Design review of the part built by this model. Coordinates are the model's own, in mm. A direction names the side the tool comes from. Coordinates: 2 decimals unless noted, no trailing zeros. Order: outer loops, then holes, each group sorted by start corner. A loop starts at its lowest first (then second) coordinate and runs counter-clockwise, first axis right, second up. Notation, with made-up numbers: (-12, -21.75) -> (44, -21.75) arc R25 cw to (44, -2.75) -> close; hole circle Ø4 at (44.25, 55.25). An arc over 180 degrees is marked (long way). Write item = value, one per line.
```python
from build123d import *

# Parameters (mm, degrees)
SKETCH1_R           = 2.75
BOSS_EXTRUDE1_DEPTH = 3.2


with BuildPart() as part:
    # Sketch1 → Boss-Extrude1 (new body)
    with BuildSketch(Plane.XY):
        Polygon((0, 82), (0, 3), (3, 0), (82, 0), (85, 3), (85, 15), (82, 18), (18, 18), (18, 82), (15, 85), (3, 85), align=None)
        with Locations((75, 9)):
            Circle(SKETCH1_R, mode=Mode.SUBTRACT)
        with Locations((47, 9)):
            Circle(SKETCH1_R, mode=Mode.SUBTRACT)
        with Locations((9, 47)):
            Circle(SKETCH1_R, mode=Mode.SUBTRACT)
        with Locations((9, 75)):
            Circle(SKETCH1_R, mode=Mode.SUBTRACT)
    extrude(amount=-BOSS_EXTRUDE1_DEPTH)


solid = part.part
```
(1) The part is to be moulded in two halves that separate along Y. For faces 3 (the cylindrical face through (8.642, 49.727, -1.578)), 4 (the cylindrical face through (8.642, 77.727, -1.578)), 5 (the flat face through (2, 84, -2)), 6 (the flat face through (83, 1, -2)), say which applies: released by +Y, released by -Y, zero draft, split by the parting line, or undercut.
Report:
face_3 = undercut
face_4 = undercut
face_5 = released by +Y
face_6 = released by -Y
(2) Insertion check: pin 1 (1.6 mm diameter, centred on y = 47.5, z = -2, fed in from +X); pin 2 (1 mm diameter, centred on x = 26.5, z = -2.5, fed in from +Y); pin 3 (1.5 mm diameter, centred on x = 22, z = -2, fed in from -Y). Each pin has a flat end and moves straight along its axis. Give the tip position at first contact, or say it passes through.
Report:
pin_1 = 18
pin_2 = 18
pin_3 = 0
(3) For faces 1 (the flat face through (50, 18, -2)), 2 (the cylindrical face through (72.253, 9.121, -1.578)), list the 3-axis set-ups (+Z, -Z, +X, -X, +Y, -Y) from which the entire face can be reached by the end or side of a thin tool; tool diameter is ignored.
Report:
face_1 = +Z, -Z, +X, +Y
face_2 = +Z, -Z
(4) We need section A-A (y = 9). Write out the cut boundary in (x, z), and give its area (3 significant figures).
Report:
outline = (0, -3.2) -> (44.25, -3.2) -> (44.25, 0) -> (0, 0) -> close; (49.75, -3.2) -> (72.25, -3.2) -> (72.25, 0) -> (49.75, 0) -> close; (77.75, -3.2) -> (85, -3.2) -> (85, 0) -> (77.75, 0) -> close
area = 237 mm²
(5) For L1, parallel to Y at x = 9, z = -1.9; L2, parallel to Y at x = 75, z = -1; L3, parallel to X at y = 78, z = -0.75, list the stretches that pass through material, from the lowest coordinate up.
Report:
L1 = 0 to 44.25, 49.75 to 72.25, 77.75 to 85
L2 = 0 to 6.25, 11.75 to 18
L3 = 0 to 18
(6) We need section D-D (y = 47). Write out the cut boundary in (x, z), and give its area (3 significant figures).
Report:
outline = (0, -3.2) -> (6.25, -3.2) -> (6.25, 0) -> (0, 0) -> close; (11.75, -3.2) -> (18, -3.2) -> (18, 0) -> (11.75, 0) -> close
area = 40.0 mm²
(7) We need section B-B (z = -0.7). Write out the cut boundary in (x, y).
Report:
outline = (0, 3) -> (3, 0) -> (82, 0) -> (85, 3) -> (85, 15) -> (82, 18) -> (18, 18) -> (18, 82) -> (15, 85) -> (3, 85) -> (0, 82) -> close; hole circle Ø5.5 at (9, 47); hole circle Ø5.5 at (9, 75); hole circle Ø5.5 at (47, 9); hole circle Ø5.5 at (75, 9)
